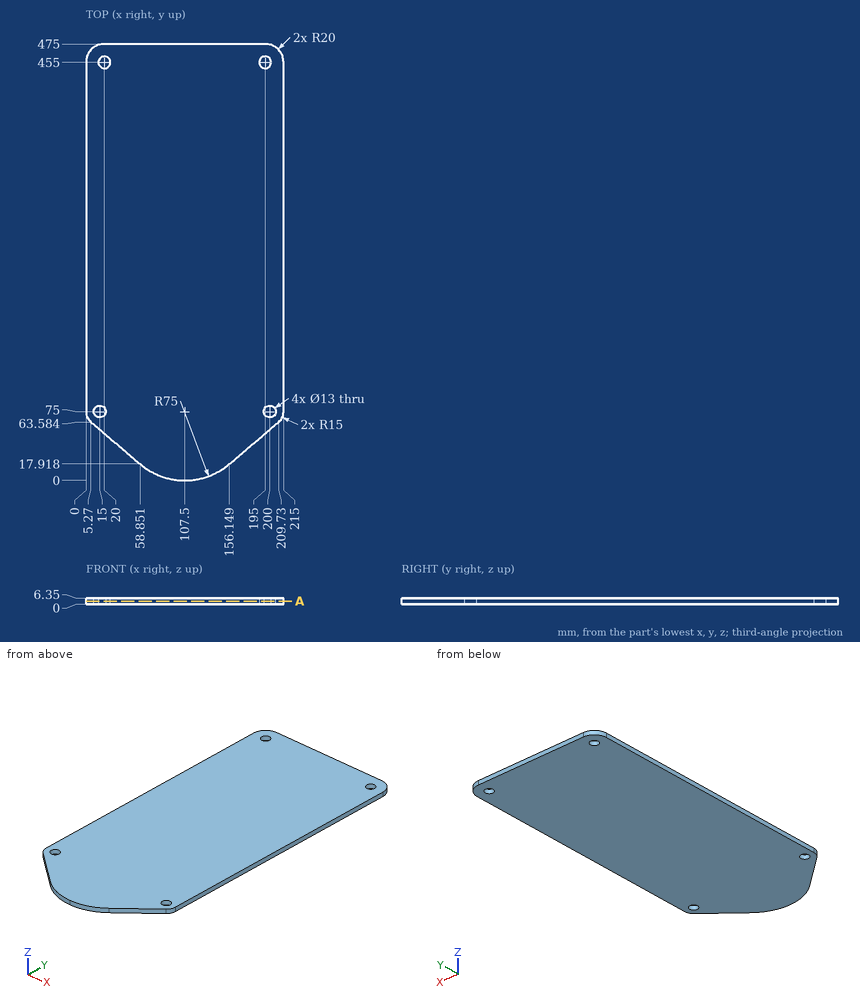
Here's the drawing with two shaded views (mm, measured from the low corner). I have some questions. Coordinates: 2 decimals unless noted, no trailing zeros. Write each loop counter-clockwise with the first axis right and the second up, starting at its lowest first coordinate (ties: lowest second). Pieces come first, ordered by that corner, then holes. Notation, with made-up numbers: (19, 60.5) -> (48, 60.5) arc R14 cw to (48, 79.5) -> close; hole circle Ø3 at (-34.5, 58.25). An arc over 180 degrees is marked (long way). Answer as CSV lines item,"result".
1) If we section it at A-A on z = 3.5: Please give me the cut outline in (x, y), then the cut area to 3 significant figures.
Check result:
outline,"(0, 75) arc R15 ccw to (5.27, 63.58) -> (58.85, 17.92) arc R75 ccw to (156.15, 17.92) -> (209.73, 63.58) arc R15 ccw to (215, 75) -> (215, 455) arc R20 ccw to (195, 475) -> (20, 475) arc R20 ccw to (0, 455) -> close; hole circle Ø13 at (15, 75); hole circle Ø13 at (20, 455); hole circle Ø13 at (195, 455); hole circle Ø13 at (200, 75)"
area,"95,800 mm²"
2) Will these pins go through, and if not, where does the flat tip stop? P1, Ø8, axis at x = 195, y = 455, coming from the -Z side (3 decimals); P2, Ø1, axis at x = 130.5, z = 1, coming from the -Y side (1 decimal); P3, Ø1.5, axis at x = 60.5, z = 1, coming from the -Y side.
Check result:
P1,"through"
P2,"y = 3.5"
P3,"y = 15.96"
3) If I drill on line 1 (X direction, y = 455, z = 2.25); line 2 (Y direction, x = 195, z = 3.25) (1 decimal); line 3 (X direction, y = 56.5, z = 3), over which ranges is the centre line in solid material (lowest first)? Write a range as from..to.
Check result:
line 1,"0..13.5, 26.5..188.5, 201.5..215"
line 2,"51..70.8, 79.2..448.5, 461.5..475"
line 3,"13.58..201.42"
